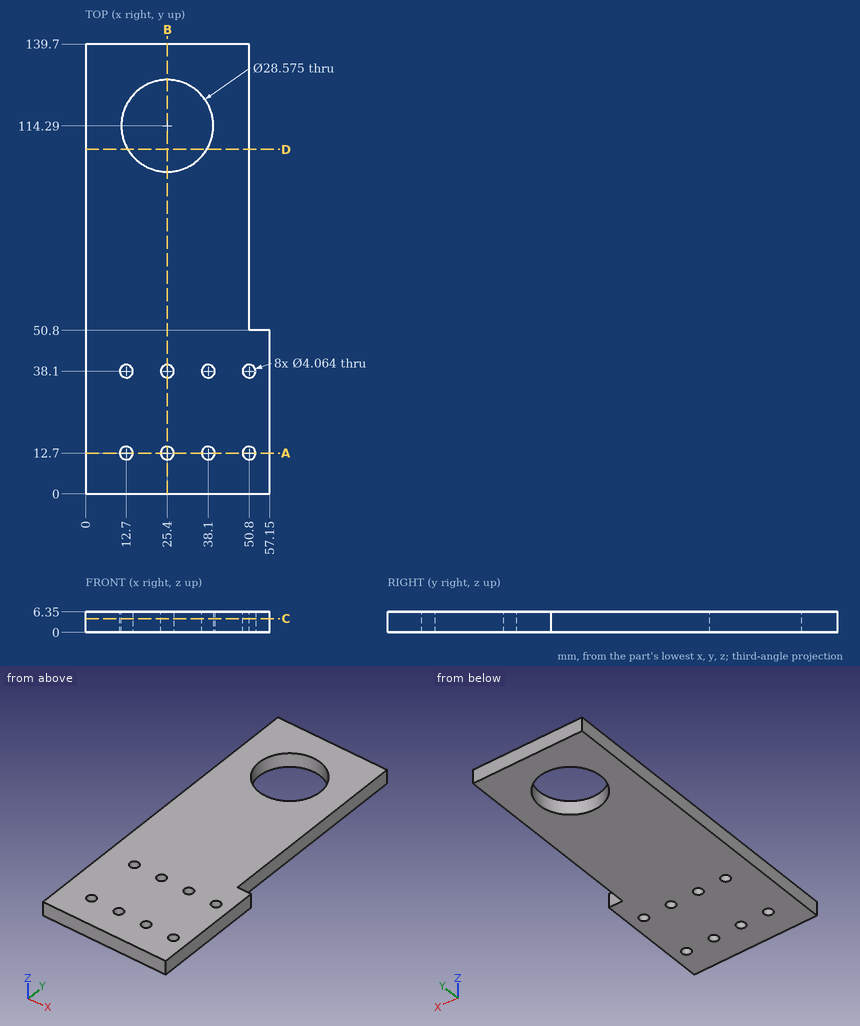
Could you check a few things on this drawing? It's one solid part, dimensions in mm from its lowest x, y, z. Give positions to 0.01 mm unless a question says otherwise; leave off trailing zeros. Order: outer loops, then holes, each group sorted by start corner. A loop starts at its lowest first (then second) coordinate and runs counter-clockwise, first axis right, second up.
1. For pin 1 (3 mm diameter, centred on y = 100.5, z = 1.5, fed in from +X); pin 2 (3.5 mm diameter, centred on x = 25.4, y = 38.1, fed in from -Z); pin 3 (1.9 mm diameter, centred on x = 53.5, z = 3, fed in from +Y), each with a flat end and sliding along its axis, tell me the tip position at first contact or that it passes through.
Answers below:
pin 1: stops at x = 50.8
pin 2: passes through
pin 3: stops at y = 50.8
2. Suppose I cut it at D-D (y = 107). Write out the boundary of the cut face in (x, z), plus the area to 3 significant figures.
Answers below:
outline: (0, 0) - (13.11, 0) - (13.11, 6.35) - (0, 6.35) - close; (37.69, 0) - (50.8, 0) - (50.8, 6.35) - (37.69, 6.35) - close
area: 167 mm2
3. Suppose I cut it at C-C (z = 4.25). State how many separate pieces and enclosed holes the cut face has, plus the area to 3 significant figures.
Answers below:
separate pieces: 1
enclosed holes: 9
area: 6,670 mm2
4. Suppose I cut it at A-A (y = 12.7). Write out the boundary of the cut face in (x, z).
Answers below:
outline: (0, 0) - (10.67, 0) - (10.67, 6.35) - (0, 6.35) - close; (14.73, 0) - (23.37, 0) - (23.37, 6.35) - (14.73, 6.35) - close; (27.43, 0) - (36.07, 0) - (36.07, 6.35) - (27.43, 6.35) - close; (40.13, 0) - (48.77, 0) - (48.77, 6.35) - (40.13, 6.35) - close; (52.83, 0) - (57.15, 0) - (57.15, 6.35) - (52.83, 6.35) - close
5. I need wall thicknesses on L1, parallel to X at y = 12.7, z = 2.5; L2, parallel to Y at x = 25.4, z = 2.25; L3, parallel to Y at x = 38, z = 3.5. Which ranges of each line are inside material? Lowest first, please.
Answers below:
L1: x = 0 to 10.67, 14.73 to 23.37, 27.43 to 36.07, 40.13 to 48.77, 52.83 to 57.15
L2: y = 0 to 10.67, 14.73 to 36.07, 40.13 to 100, 128.58 to 139.7
L3: y = 0 to 10.67, 14.73 to 36.07, 40.13 to 107.55, 121.03 to 139.7
6. Suppose I cut it at B-B (x = 25.4). Write out the boundary of the cut face in (y, z), plus the area to 3 significant figures.
Answers below:
outline: (0, 0) - (10.67, 0) - (10.67, 6.35) - (0, 6.35) - close; (14.73, 0) - (36.07, 0) - (36.07, 6.35) - (14.73, 6.35) - close; (40.13, 0) - (100, 0) - (100, 6.35) - (40.13, 6.35) - close; (128.58, 0) - (139.7, 0) - (139.7, 6.35) - (128.58, 6.35) - close
area: 654 mm2
